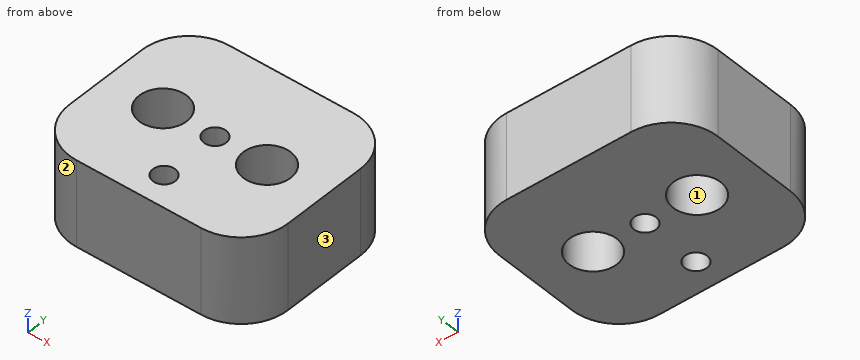
```python
from build123d import *

# Parameters (mm, degrees)
SKETCH1_W                = 14.732
SKETCH1_H                = 12.0904
BOSS_EXTRUDE1_DEPTH      = 5.8
SKETCH2_R                = 0.75
CUT_EXTRUDE1_DEPTH       = 5.8
M3_CLEARANCE_HOLE1_D     = 3.2
M3_CLEARANCE_HOLE1_DEPTH = 36.28
M3_CLEARANCE_HOLE1_TIP   = 0.96137699
FILLET1_R                = 3.175


with BuildPart() as part:
    # Sketch1 → Boss-Extrude1 (new body)
    with BuildSketch(Plane.XY):
        with Locations((7.366, 6.0452)):
            Rectangle(SKETCH1_W, SKETCH1_H)
    extrude(amount=BOSS_EXTRUDE1_DEPTH)

    # Sketch2 → Cut-Extrude1 (cut)
    with BuildSketch(Plane.XY.offset(5.8)):
        with Locations((7.366, 6.0452)):
            Circle(SKETCH2_R)
        with Locations((7.366, 2)):
            Circle(SKETCH2_R)
    extrude(amount=-CUT_EXTRUDE1_DEPTH, mode=Mode.SUBTRACT)

    # M3 Clearance Hole1
    with Locations(Plane.XY.offset(5.8)):
        with Locations((3.8608, 6.0452), (10.8712, 6.0452)):
            Hole(M3_CLEARANCE_HOLE1_D / 2, depth=M3_CLEARANCE_HOLE1_DEPTH)
            with Locations((0, 0, -(M3_CLEARANCE_HOLE1_DEPTH + M3_CLEARANCE_HOLE1_TIP / 2))):  # 118° drill point
                Cone(0, M3_CLEARANCE_HOLE1_D / 2, M3_CLEARANCE_HOLE1_TIP, mode=Mode.SUBTRACT)

    # Fillet1
    fillet1_edges = [part.edges().sort_by_distance(p)[0] for p in [
        (0, 12.0904, 2.9),
        (14.732, 12.0904, 2.9),
        (14.732, 0, 2.9),
        (0, 0, 2.9),
    ]]
    fillet(fillet1_edges, radius=FILLET1_R)


solid = part.part
```
Here's how the part is built. I have some questions about the finished solid (model axes, mm). Face numbers are marked on the shaded views. Coordinates: 2 decimals unless noted, no trailing zeros. Order: outer loops, then holes, each group sorted by start corner. A loop starts at its lowest first (then second) coordinate and runs counter-clockwise, first axis right, second up. Notation, with made-up numbers: M 49.25,81.5 L 108.25,81.5 A23 ccw 108.25,106.5 Z; hole C 57.5,27.5 d10. An arc over 180 degrees is marked long. Answer as a JSON object with one key per item and string values. Group by question number.
(1) Suppose I cut it at C-C, the plane z = 1.2. Please give me the cut outline in (x, y) (3 decimals), then the cut area to 3 significant figures.
(2) Suppose I cut it at D-D, the plane y = 2. Please give me the cut outline in (x, z).
(3) For pin 1 (1.5 mm diameter, centred on y = 10.5, z = 1.5, fed in from +X), with a flat end and sliding along its axis, tell me the tip position at first contact or that it passes through.
(4) Suppose I cut it at B-B, the plane y = 5. Please give me the cut outline in (x, z).
(5) I need wall thicknesses on probe 1 along X at (y, z) = (6.25, 2.45); probe 2 along X at (y, z) = (7, 3.55); probe 3 along Y at (x, z) = (4.5, 4.3). Which ranges of each line are inside material? Lowest first, please.
(6) If we mould it in two halves opening along Y, with no side actions, what happens to the marked faces 1, 2 and 3? For each: released by +Y, released by -Y, zero draft, split by the parting line, or undercut.
(7) Suppose I cut it at A-A, the plane x = 12.25. Please give me the cut outline in (y, z), then the cut area to 3 significant figures.
Values found:
{
 "1": {"outline": "M 0,3.175 A3.175 ccw 3.175,0 L 11.557,0 A3.175 ccw 14.732,3.175 L 14.732,8.915 A3.175 ccw 11.557,12.09 L 3.175,12.09 A3.175 ccw 0,8.915 Z; hole C 3.861,6.045 d3.2; hole C 7.366,2 d1.5; hole C 7.366,6.045 d1.5; hole C 10.871,6.045 d3.2", "area": "150 mm^2"},
 "2": {"outline": "M 0.23,0 L 6.62,0 L 6.62,5.8 L 0.23,5.8 Z; M 8.12,0 L 14.51,0 L 14.51,5.8 L 8.12,5.8 Z"},
 "3": {"pin 1": "stops at x = 14.62"},
 "4": {"outline": "M 0,0 L 2.65,0 L 2.65,5.8 L 0,5.8 Z; M 5.07,0 L 9.66,0 L 9.66,5.8 L 5.07,5.8 Z; M 12.08,0 L 14.73,0 L 14.73,5.8 L 12.08,5.8 Z"},
 "5": {"probe 1": "x = 0 to 2.27, 5.45 to 6.64, 8.09 to 9.28, 12.46 to 14.73", "probe 2": "x = 0 to 2.58, 5.14 to 9.59, 12.16 to 14.73", "probe 3": "y = 0 to 4.58, 7.51 to 12.09"},
 "6": {"face 1": "undercut", "face 2": "released by -Y", "face 3": "zero draft"},
 "7": {"outline": "M 0.08,0 L 5.23,0 L 5.23,5.8 L 0.08,5.8 Z; M 6.86,0 L 12.01,0 L 12.01,5.8 L 6.86,5.8 Z", "area": "59.8 mm^2"}
}
